```python
from build123d import *

# Parameters (mm, degrees)
SKETCH1_W                        = 250
SKETCH1_H                        = 344
SKETCH1_R                        = 23.5
SKETCH1_R_2                      = 8.5
SKETCH1_R_3                      = 12.5
BOSS_EXTRUDE1_DEPTH              = 12
TAP_DRILL_FOR_M5_TAP1_AT_2_COUNT = 2
TAP_DRILL_FOR_M5_TAP1_AT_2_PITCH = 46
TAP_DRILL_FOR_M6_TAP1_D          = 5
TAP_DRILL_FOR_M5_TAP2_D          = 4.2
TAP_DRILL_FOR_M5_TAP2_DEPTH      = 15
TAP_DRILL_FOR_M5_TAP2_TIP        = 1.2618073
TAP_DRILL_FOR_M5_TAP3_AT_2_COUNT = 2
TAP_DRILL_FOR_M5_TAP3_AT_2_PITCH = 55
TAP_DRILL_FOR_M5_TAP3_AT_3_COUNT = 2
TAP_DRILL_FOR_M5_TAP3_AT_3_PITCH = 110


with BuildPart() as part:
    # Sketch1 → Boss-Extrude1 (new body)
    with BuildSketch(Plane.XY):
        with Locations((0, 122)):
            Rectangle(SKETCH1_W, SKETCH1_H)
        with Locations((-80, 244)):
            Circle(SKETCH1_R, mode=Mode.SUBTRACT)
        with Locations((80, 244)):
            Circle(SKETCH1_R, mode=Mode.SUBTRACT)
        with Locations((-100, 83)):
            Circle(SKETCH1_R_2, mode=Mode.SUBTRACT)
        with Locations((100, 83)):
            Circle(SKETCH1_R_2, mode=Mode.SUBTRACT)
        with Locations((-30, 0)):
            Circle(SKETCH1_R_3, mode=Mode.SUBTRACT)
        with Locations((85, 0)):
            Circle(SKETCH1_R_3, mode=Mode.SUBTRACT)
    extrude(amount=BOSS_EXTRUDE1_DEPTH)

    # Sketch5 → Tap Drill for M5 Tap1 (revolve, cut)
    with BuildSketch(Plane(origin=(-125, 282, 6), x_dir=(0, 0, 1), z_dir=(0, 1, 0))):
        Polygon((0, 0), (0, 16.2618073), (2.1, 15), (2.1, 0), align=None)
    tap_drill_for_m5_tap1 = revolve(axis=Axis((-131.35, 282, 6), (1, 0, 0)), mode=Mode.SUBTRACT)

    # Tap Drill for M5 Tap1 at 2: Tap Drill for M5 Tap1 ×2
    with Locations(*[(0, -i * TAP_DRILL_FOR_M5_TAP1_AT_2_PITCH, 0) for i in range(1, TAP_DRILL_FOR_M5_TAP1_AT_2_COUNT)]):
        add(tap_drill_for_m5_tap1, mode=Mode.SUBTRACT)

    # Mirror1: Tap Drill for M5 Tap1 across plane
    add(tap_drill_for_m5_tap1.mirror(Plane(origin=(0, 0, 0), x_dir=(0, 0, 1), z_dir=(1, 0, 0))), mode=Mode.SUBTRACT)

    # Mirror1 copy 1 sketch → Mirror1 copy 1 (revolve, cut)
    with BuildSketch(Plane(origin=(125, 236, 6), x_dir=(0, 0, 1), z_dir=(0, 1, 0))):
        Polygon((0, 0), (0, -16.2618073), (2.1, -15), (2.1, 0), align=None)
    revolve(axis=Axis((131.35, 236, 6), (1, 0, 0)), mode=Mode.SUBTRACT)

    # Tap Drill for M6 Tap1 (through all)
    with Locations(Plane.XY.offset(12)):
        with Locations((-105, 269), (-55, 269), (-55, 219), (-105, 219), (55, 219), (105, 219), (105, 269), (55, 269), (-55, 25), (-5, 25), (-5, -25), (-55, -25), (60, 25), (110, 25), (110, -25), (60, -25)):
            Hole(TAP_DRILL_FOR_M6_TAP1_D / 2)

    # Tap Drill for M5 Tap2
    with Locations(Plane(origin=(0, -50, 0), x_dir=(-1, 0, 0), z_dir=(0, -1, 0))):
        with Locations((-113, -6), (-67, -6), (67, -6), (113, -6)):
            Hole(TAP_DRILL_FOR_M5_TAP2_D / 2, depth=TAP_DRILL_FOR_M5_TAP2_DEPTH)
            with Locations((0, 0, -(TAP_DRILL_FOR_M5_TAP2_DEPTH + TAP_DRILL_FOR_M5_TAP2_TIP / 2))):  # 118° drill point
                Cone(0, TAP_DRILL_FOR_M5_TAP2_D / 2, TAP_DRILL_FOR_M5_TAP2_TIP, mode=Mode.SUBTRACT)

    # Sketch19 → Tap Drill for M5 Tap3 (revolve, cut)
    with BuildSketch(Plane(origin=(125, 97, 6), x_dir=(0, 0, -1), z_dir=(0, 1, 0))):
        Polygon((0, 0), (0, 11.2618073), (2.1, 10), (2.1, 0), align=None)
    tap_drill_for_m5_tap3 = revolve(axis=Axis((131.35, 97, 6), (-1, 0, 0)), mode=Mode.SUBTRACT)

    # Tap Drill for M5 Tap3 at 2: Tap Drill for M5 Tap3 ×2
    with Locations(*[(0, i * TAP_DRILL_FOR_M5_TAP3_AT_2_PITCH, 0) for i in range(1, TAP_DRILL_FOR_M5_TAP3_AT_2_COUNT)]):
        add(tap_drill_for_m5_tap3, mode=Mode.SUBTRACT)

    # Tap Drill for M5 Tap3 at 3: Tap Drill for M5 Tap3 ×2
    with Locations(*[(0, i * TAP_DRILL_FOR_M5_TAP3_AT_3_PITCH, 0) for i in range(1, TAP_DRILL_FOR_M5_TAP3_AT_3_COUNT)]):
        add(tap_drill_for_m5_tap3, mode=Mode.SUBTRACT)

    # Mirror2: Tap Drill for M5 Tap3 across plane
    add(tap_drill_for_m5_tap3.mirror(Plane(origin=(0, 0, 0), x_dir=(0, 0, 1), z_dir=(1, 0, 0))), mode=Mode.SUBTRACT)

    # Mirror2 copy 1 sketch → Mirror2 copy 1 (revolve, cut)
    with BuildSketch(Plane(origin=(-125, 152, 6), x_dir=(0, 0, -1), z_dir=(0, 1, 0))):
        Polygon((0, 0), (0, -11.2618073), (2.1, -10), (2.1, 0), align=None)
    revolve(axis=Axis((-131.35, 152, 6), (-1, 0, 0)), mode=Mode.SUBTRACT)

    # Mirror2 copy 2 sketch → Mirror2 copy 2 (revolve, cut)
    with BuildSketch(Plane(origin=(-125, 207, 6), x_dir=(0, 0, -1), z_dir=(0, 1, 0))):
        Polygon((0, 0), (0, -11.2618073), (2.1, -10), (2.1, 0), align=None)
    revolve(axis=Axis((-131.35, 207, 6), (-1, 0, 0)), mode=Mode.SUBTRACT)


solid = part.part
```
Geometry: final body of the model. Coordinates: model frame, mm. Coordinates: 2 decimals unless noted, no trailing zeros. Order: outer loops, then holes, each group sorted by start corner. A loop starts at its lowest first (then second) coordinate and runs counter-clockwise, first axis right, second up. Notation, with made-up numbers: (31.25, 4.25) -> (54.25, 4.25) arc R17 ccw to (54.25, 19.25) -> close; hole circle Ø9 at (81.5, 60). An arc over 180 degrees is marked (long way). Use CSV: the item, a comma, the result in double quotes.
1) Section C-C on y = 86.5. Output: boundary loops of the cut face in (x, z).
Findings:
outline,"(-125, 0) -> (-107.75, 0) -> (-107.75, 12) -> (-125, 12) -> close; (-92.25, 0) -> (92.25, 0) -> (92.25, 12) -> (-92.25, 12) -> close; (107.75, 0) -> (125, 0) -> (125, 12) -> (107.75, 12) -> close"
2) Section B-B on x = -95.5. Output: boundary loops of the cut face in (y, z), then the cut area to 3 significant figures.
Findings:
outline,"(-50, 0) -> (75.79, 0) -> (75.79, 12) -> (-50, 12) -> close; (90.21, 0) -> (226.34, 0) -> (226.34, 12) -> (90.21, 12) -> close; (261.66, 0) -> (294, 0) -> (294, 12) -> (261.66, 12) -> close"
area,"3,530 mm^2"
3) Line query: line 1 (Y direction, x = 122.5, z = 6); line 2 (Y direction, x = -87, z = 4); line 3 (Z direction, x = 118, y = 207). Output: solid intervals per line, ascending.
Findings:
line 1,"y = -50 to 94.9, 99.1 to 149.9, 154.1 to 204.9, 209.1 to 233.9, 238.1 to 279.9, 284.1 to 294"
line 2,"y = -50 to 221.57, 266.43 to 294"
line 3,"z = 0 to 3.9, 8.1 to 12"
4) Mould query, pull axis X, two halves, no side actions, for faces 1 (the flat face through (-2, 124, 0)), 2 (the cylindrical face through (-108.49, 83.37, 5.92)), 3 (the flat face through (-125, 120, 6)), 4 (the cylindrical face through (96.923, 3.755, 5.916)). Classes: +X half, -X half, draft (parallel to the pull), parting line (faces both ways), or undercut.
Findings:
face 1,"draft"
face 2,"undercut"
face 3,"-X half"
face 4,"undercut"
5) Pin query (flat end, axial travel): pin 1 Ø4 at (y, z) = (282, 6) entering from -X; pin 2 Ø4 at (y, z) = (207, 6) entering from -X. Return the tip coordinate at first contact, or that it passes through.
Findings:
pin 1,"stops at x = -109.94"
pin 2,"stops at x = -114.94"
6) Section A-A on x = -33.5. Output: boundary loops of the cut face in (y, z), then the cut area to 3 significant figures.
Findings:
outline,"(-50, 0) -> (-12, 0) -> (-12, 12) -> (-50, 12) -> close; (12, 0) -> (294, 0) -> (294, 12) -> (12, 12) -> close"
area,"3,840 mm^2"
